Geometry: final body of the model. Coordinates: model frame, mm. A direction names the side the tool comes from. Coordinates: 2 decimals unless noted, no trailing zeros. Write each loop counter-clockwise with the first axis right and the second up, starting at its lowest first coordinate (ties: lowest second). Pieces come first, ordered by that corner, then holes. Notation, with made-up numbers: (59.5, 38.5) - (73.5, 38.5) arc R22 cw to (73.5, 75.5) - close; hole circle Ø4 at (-18, 85). An arc over 180 degrees is marked (long way). Answer as a JSON object with one key per item and string values. Group by question number.
Item 1: First-contact query: pin 1 Ø3 at (x, z) = (1.5, 4.5) entering from +Y; pin 2 Ø2.5 at (x, y) = (7.5, 7.5) entering from +Z; pin 3 Ø1.9 at (x, z) = (2, 3) entering from -Y; pin 4 Ø10 at (x, y) = (20.5, 15.5) entering from +Z. Flat tips, straight axial feed; report the tip coordinate or a pass-through.
Item 2: Section A-A on x = 7.5. Return loops of the section in (y, z).
Item 3: Section C-C on z = 1.5. Return loops of the section in (x, y), and give its area (3 significant figures).
Item 4: Section D-D on y = 17.25. Return loops of the section in (x, z).
Item 5: Section B-B on y = 7.5. Return loops of the section in (x, z), and give its area (3 significant figures).
Item 6: Line query: line 1 along Y through (x, z) = (7.5, 2.5); line 2 along Y through (x, z) = (18.5, 5.5); line 3 along X through (y, z) = (16.5, 2). Output: solid intervals per line, ascending. Write a range as from..to.
Item 7: Mould query, pull axis Y, two halves, no side actions, for faces 1 (the flat face through (2, 0, 3)), 2 (the flat face through (3.75, 18, 3)), 3 (the cylindrical face through (7.15, 9.06, 3.32)). Classes: pulls with the +Y half, pulls with the -Y half, needs draft (parallel to the pull), parting line crosses it, or undercut.
Item 8: Set-up query: faces 4 (the flat face through (17, 0, 3)), 5 (the flat face through (18, 5, 3)), 6 (the flat face through (3.75, -2, 3)), 7 (the flat face through (18, 15, 3)). Return all of +Z, -Z, +X, -X, +Y, -Y with unobstructed straight access to the full face (end or side cutting, diameter ignored); none if empty.
Autodesk Inventor part; units mm, degrees
ref_plane "YZ Plane" through (0, 0, 0) normal (1, 0, 0) x (0, 1, 0)
ref_plane "XZ Plane" through (0, 0, 0) normal (0, 1, 0) x (-1, 0, 0)
ref_plane "XY Plane" through (0, 0, 0) normal (0, 0, 1) x (1, 0, 0)
sketch "Sketch1" plane through (0, 0, 0) normal (0, 0, 1) x (1, 0, 0)
  line L0 (0, 0) -> (3.75, 0)
  line L1 (3.75, 0) -> (3.75, -5)
  line L2 (3.75, -5) -> (11.25, -5)
  line L3 (11.25, -5) -> (11.25, 0)
  line L4 (11.25, 0) -> (23.75, 0)
  line L5 (23.75, 0) -> (23.75, 15)
  line L6 (23.75, 15) -> (11.25, 15)
  line L7 (11.25, 15) -> (11.25, 20)
  line L8 (11.25, 20) -> (3.75, 20)
  line L9 (3.75, 20) -> (3.75, 15)
  line L10 (3.75, 15) -> (0, 15)
  line L11 (0, 15) -> (0, 0)
  line L12 (21.731, 10) -> (15, 10)
  line L13 (15, 10) -> (15, 5)
  line L14 (15, 5) -> (21.731, 5)
  line L15 (21.731, 5) -> (21.731, 10)
  circle A0 centre (7.5, 7.5) radius 1.6
  point P0 (21.731, 7.5)
  point P1 (23.75, 7.5)
  point P2 (7.5, -5)
  point P3 (0, 7.5)
  dimension "d0" = 15
  dimension "d1" = 3.75
  dimension "d2" = 5
  dimension "d3" = 7.5
  dimension "d4" = 12.5
  dimension "d5" = 6.731
  dimension "d6" = 5
  dimension "d7" = 3.75
  dimension "d12" = 3.2
extrude "Extrusion1" add sketch "Sketch1" along normal blind 6.731
equation "\"d5\" = THICKB"
equation "\"d7\" = d1"
equation "\"d8\" = THICKB"
equation "\"THICKA\" = 3.175"
equation "\"THICKB\" = 6.731"
equation "\"THICKC\" = 12.7"
equation "\"MAGDIA\" = 9.5"
equation "\"BALLDIA\" = 12"
equation "\"THICKPLY\" = 5"
properties part number "Frame_Upper_Vertical_Plate_A"
Checks:
{
 "1": {"pin 1": "y = 15", "pin 2": "through", "pin 3": "y = 0", "pin 4": "z = 6.73"},
 "2": {"outline": "(-5, 0) - (5.9, 0) - (5.9, 6.73) - (-5, 6.73) - close; (9.1, 0) - (20, 0) - (20, 6.73) - (9.1, 6.73) - close"},
 "3": {"outline": "(0, 0) - (3.75, 0) - (3.75, -5) - (11.25, -5) - (11.25, 0) - (23.75, 0) - (23.75, 15) - (11.25, 15) - (11.25, 20) - (3.75, 20) - (3.75, 15) - (0, 15) - close; hole circle Ø3.2 at (7.5, 7.5); hole (15, 5) - (21.73, 5) - (21.73, 10) - (15, 10) - close", "area": "390 mm^2"},
 "4": {"outline": "(3.75, 0) - (11.25, 0) - (11.25, 6.73) - (3.75, 6.73) - close"},
 "5": {"outline": "(0, 0) - (5.9, 0) - (5.9, 6.73) - (0, 6.73) - close; (9.1, 0) - (15, 0) - (15, 6.73) - (9.1, 6.73) - close; (21.73, 0) - (23.75, 0) - (23.75, 6.73) - (21.73, 6.73) - close", "area": "93.0 mm^2"},
 "6": {"line 1": "-5..5.9, 9.1..20", "line 2": "0..5, 10..15", "line 3": "3.75..11.25"},
 "7": {"face 1": "pulls with the -Y half", "face 2": "needs draft", "face 3": "undercut"},
 "8": {"face 4": "+Z, -Z, +X, -Y", "face 5": "+Z, -Z", "face 6": "+Z, -Z, -X, -Y", "face 7": "+Z, -Z, +X, +Y"}
}
